Here's the drawing with two shaded views (mm, measured from the low corner). I have some questions. Give positions to 0.01 mm unless a question says otherwise; leave off trailing zeros. Loops run counter-clockwise (first coordinate to the right, second up) from the corner with the lowest first, then second, coordinate; pieces in that order, holes last.
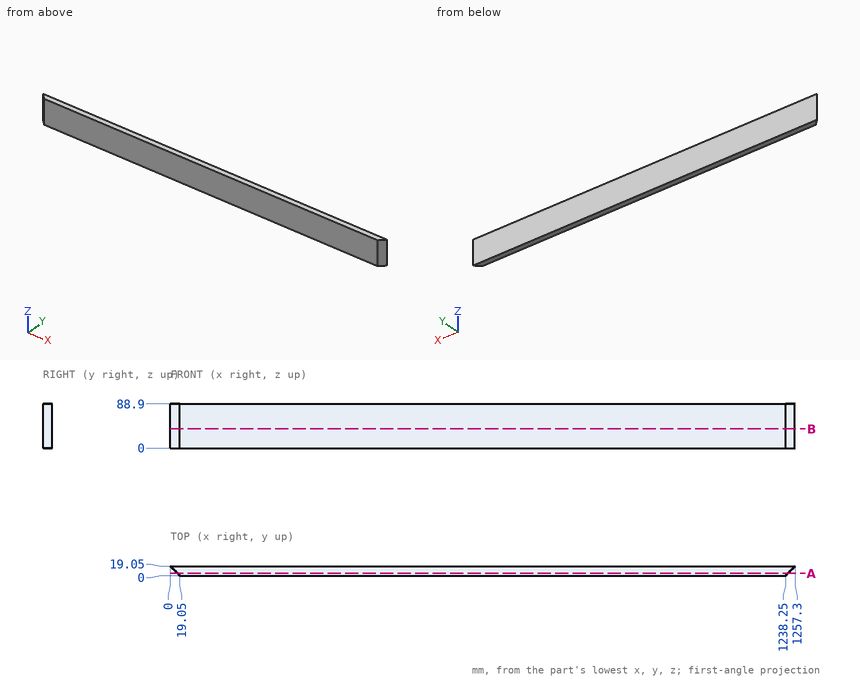
(1) Please list where these lines run through material, in increasing order: probe 1 along X at (y, z) = (6.25, 61); probe 2 along X at (y, z) = (14.75, 66.5).
Returned:
probe 1: x = 12.8 to 1244.5
probe 2: x = 4.3 to 1253
(2) Suppose I cut it at B-B on z = 39. List the corners of the cut face in (x, y) for me.
Returned:
outline: (0, 19.05) - (19.05, 0) - (1238.25, 0) - (1257.3, 19.05) - close
(3) Suppose I cut it at A-A on y = 4.5. List the corners of the cut face in (x, z) for me.
Returned:
outline: (14.55, 0) - (1242.75, 0) - (1242.75, 88.9) - (14.55, 88.9) - close
(4) Will these pins go through, and if not, where does the flat tip stop? P1, Ø3, axis at y = 4.5, z = 28, coming from the +X side; P2, Ø3, axis at y = 12, z = 63, coming from the -X side; P3, Ø8, axis at y = 8, z = 49, coming from the -X side.
Returned:
P1: stops at x = 1244.25
P2: stops at x = 5.55
P3: stops at x = 7.05
